The model under review builds one solid part; all positions refer to its coordinate system, in mm. Face numbers are marked on the shaded views. A direction names the side the tool comes from. Coordinates: 2 decimals unless noted, no trailing zeros. Write each loop counter-clockwise with the first axis right and the second up, starting at its lowest first coordinate (ties: lowest second). Pieces come first, ordered by that corner, then holes.
1) Add section C-C, the plane y = -11. State the section outline as (x, z) points, then the cut area to 3 significant figures.
2) For P1, Ø9.5, axis at x = 0, z = 0, coming from the +Y side; P2, Ø1.3, axis at y = 1, z = -19, coming from the +X side; P3, Ø1.3, axis at x = 21, y = -56.5, coming from the +Z side; P4, Ø2, axis at x = -17.5, y = 1.5, coming from the -Z side, all flat-tipped, find the tip position at first contact; note any pin that passes through.
3) For line 1 (Z direction, x = 0, y = 1); line 2 (X direction, y = -56.45, z = 0); line 3 (X direction, y = 2.9, z = -12.5), list the stretches that pass through material, from the lowest coordinate up.
4) Mouldability with a two-part tool opening along X and no side actions: class the marked faces 3 and 4 as released by +X, released by -X, zero draft, split by the parting line, or undercut.
5) Machinability: for the marked faces 1 and 2, which of the approach directions +Z, -Z, +X, -X, +Y, -Y give a long, thin tool a straight path to every point of the face, cutting with its end or side? Answer none if there is none.
6) Add section D-D, the plane z = 0. Give the number of separate pieces and of enclosed holes in the cut face, then the cut area to 3 significant figures.
7) Add section B-B, the plane x = -14. State the section outline as (y, z) points, then the cut area to 3 significant figures.
8) Add section A-A, the plane z = 12.5. State the section outline as (x, y) points.
from build123d import *

# Parameters (mm, degrees)
BOSS_EXTRUDE1_DEPTH      = 4.5
SKETCH2_R                = 6
SKETCH2_R_2              = 2
SKETCH2_R_3              = 3.5
CUT_EXTRUDE1_DEPTH       = 5.5
FILLET1_R                = 5
SKETCH4_R                = 3.5
BOSS_EXTRUDE2_DEPTH      = 27.5
BOSS_EXTRUDE2_DEPTH_BACK = 4.5


with BuildPart() as part:
    # Sketch1 → Boss-Extrude1 (new body)
    with BuildSketch(Plane(origin=(0, 0, 0), x_dir=(1, 0, 0), z_dir=(0, 1, 0))):
        with BuildLine():
            Line((4.5, 29), (4.5, -29))
            ThreePointArc((4.5, -29), (0, -33.5), (-4.5, -29))
            Line((-4.5, -29), (-4.5, 29))
            ThreePointArc((-4.5, 29), (0, 33.5), (4.5, 29))
        make_face()
        with BuildLine():
            Line((29, -4.5), (-29, -4.5))
            ThreePointArc((-29, -4.5), (-33.5, 0), (-29, 4.5))
            Line((-29, 4.5), (29, 4.5))
            ThreePointArc((29, 4.5), (33.5, 0), (29, -4.5))
        make_face()
    extrude(amount=BOSS_EXTRUDE1_DEPTH)

    # Sketch2 → Cut-Extrude1 (cut, through all)
    with BuildSketch(Plane(origin=(0, 4.5, 0), x_dir=(1, 0, 0), z_dir=(0, 1, 0))):
        Circle(SKETCH2_R)
        with Locations((9.5, 0)):
            Circle(SKETCH2_R_2)
        with Locations((29, 0)):
            Circle(SKETCH2_R_3)
        with Locations((0, 12.5)):
            Circle(SKETCH2_R_2)
        with Locations((0, -29)):
            Circle(SKETCH2_R_3)
        with Locations((-29, 0)):
            Circle(SKETCH2_R_3)
        with Locations((0, 29)):
            Circle(SKETCH2_R_3)
        with Locations((-9.5, 0)):
            Circle(SKETCH2_R_2)
        with Locations((0, -12.5)):
            Circle(SKETCH2_R_2)
    extrude(amount=-CUT_EXTRUDE1_DEPTH, mode=Mode.SUBTRACT)

    # Fillet1
    fillet1_edges = [part.edges().sort_by_distance(p)[0] for p in [
        (4.5, 2.25, -4.5),
        (4.5, 2.25, 4.5),
        (-4.5, 2.25, -4.5),
        (-4.5, 2.25, 4.5),
    ]]
    fillet(fillet1_edges, radius=FILLET1_R)

    # Sketch4 → Boss-Extrude2 (add, two sides)
    with BuildSketch(Plane.XZ) as boss_extrude2_sk:
        with Locations((0, -29)):
            Circle(SKETCH4_R)
        with Locations((-29, 0)):
            Circle(SKETCH4_R)
        with Locations((0, 29)):
            Circle(SKETCH4_R)
        with Locations((29, 0)):
            Circle(SKETCH4_R)
    extrude(amount=BOSS_EXTRUDE2_DEPTH)
    extrude(boss_extrude2_sk.sketch, amount=-BOSS_EXTRUDE2_DEPTH_BACK)

    # Mirror2: part across plane


with BuildPart() as part_1:
    add(part.part)
    add(part.part.mirror(Plane(origin=(0, -27.5, 29), x_dir=(0, 0, 1), z_dir=(0, -1, 0))))


solid = part_1.part
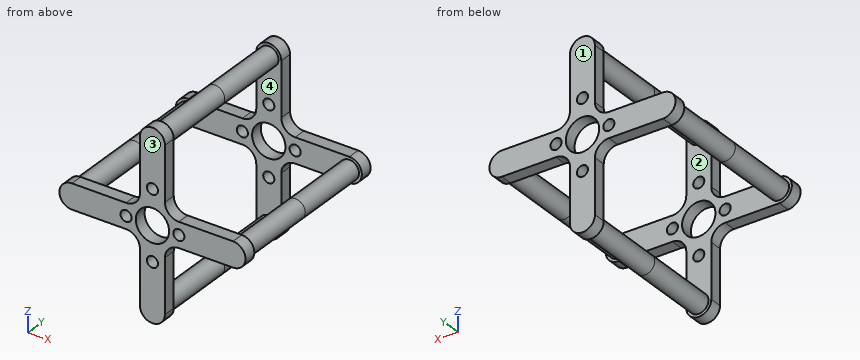
Geometry results:
1. outline: circle Ø7 at (-29, 0); circle Ø7 at (0, -29); circle Ø7 at (0, 29); circle Ø7 at (29, 0)
1. area: 154 mm2
2. P1: passes through
2. P2: stops at x = 4.5
2. P3: stops at z = 4.5
2. P4: stops at z = -4.5
3. line 1: z = -33.5 to -14.5, -10.5 to -6, 6 to 10.5, 14.5 to 33.5
3. line 2: x = -33.5 to -11.5, -7.5 to -6, 6 to 7.5, 11.5 to 33.5
3. line 3: x = -4.5 to -2, 2 to 4.5
4. face 3: zero draft
4. face 4: undercut
5. face 1: +Z, -Z, +X, -X, +Y
5. face 2: none
6. separate pieces: 6
6. enclosed holes: 0
6. area: 1,190 mm2
7. outline: (-59.5, -4.5) - (-55, -4.5) - (-55, 4.5) - (-59.5, 4.5) - close; (0, -4.5) - (4.5, -4.5) - (4.5, 4.5) - (0, 4.5) - close
7. area: 81.0 mm2
8. outline: (-4.5, -59.5) - (-2, -59.5) - (-2, -55) - (-4.5, -55) - close; (-4.5, 0) - (-2, 0) - (-2, 4.5) - (-4.5, 4.5) - close; (2, -59.5) - (4.5, -59.5) - (4.5, -55) - (2, -55) - close; (2, 0) - (4.5, 0) - (4.5, 4.5) - (2, 4.5) - close
